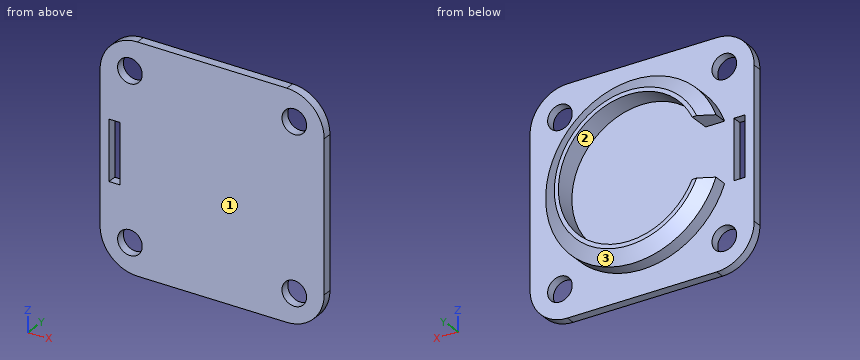
from build123d import *

# Parameters (mm, degrees)
SKETCH2_R           = 11.75
BOSS_EXTRUDE1_DEPTH = 4
CUT_EXTRUDE1_DEPTH  = 4
SKETCH4_W           = 30
SKETCH4_H           = 30
SKETCH4_R           = 1.65
BOSS_EXTRUDE2_DEPTH = 1.2
FILLET2_R           = 5
SKETCH6_W           = 1.5
SKETCH6_H           = 8
CUT_EXTRUDE2_DEPTH  = 10
CHAMFER1_SIZE       = 1
CHAMFER1_SIZE2      = 1.804047755


with BuildPart() as part:
    # Sketch2 → Boss-Extrude1 (new body)
    with BuildSketch(Plane(origin=(0, 0, 0), x_dir=(1, 0, 0), z_dir=(0, 1, 0))):
        with Locations(Location((0, 0, 0), (0, 0, 270))):
            Circle(SKETCH2_R)
    extrude(amount=BOSS_EXTRUDE1_DEPTH)

    # Sketch3 → Cut-Extrude1 (cut)
    with BuildSketch(Plane(origin=(0, 4, 0), x_dir=(1, 0, 0), z_dir=(0, 1, 0))):
        with BuildLine():
            Line((-8.506468127, 4), (-15.473450434, 4))
            Line((-15.473450434, 4), (-15.473450434, -4))
            Line((-15.473450434, -4), (-8.506468127, -4))
            ThreePointArc((-8.506468127, -4), (9.4, 0), (-8.506468127, 4))
        make_face()
    extrude(amount=-CUT_EXTRUDE1_DEPTH, mode=Mode.SUBTRACT)

    # Sketch4 → Boss-Extrude2 (add)
    with BuildSketch(Plane(origin=(0, 0, 0), x_dir=(1, 0, 0), z_dir=(0, 1, 0))):
        Rectangle(SKETCH4_W, SKETCH4_H)
        with Locations(Location((11, -11, 0), (0, 0, 270))):
            Circle(SKETCH4_R, mode=Mode.SUBTRACT)
        with Locations(Location((-11, -11, 0), (0, 0, 270))):
            Circle(SKETCH4_R, mode=Mode.SUBTRACT)
        with Locations(Location((-11, 11, 0), (0, 0, 270))):
            Circle(SKETCH4_R, mode=Mode.SUBTRACT)
        with Locations(Location((11, 11, 0), (0, 0, 270))):
            Circle(SKETCH4_R, mode=Mode.SUBTRACT)
    extrude(amount=BOSS_EXTRUDE2_DEPTH)

    # Fillet2
    fillet2_edges = [part.edges().sort_by_distance(p)[0] for p in [
        (15, 0.6, 15),
        (15, 0.6, -15),
        (-15, 0.6, -15),
        (-15, 0.6, 15),
    ]]
    fillet(fillet2_edges, radius=FILLET2_R)

    # Sketch6 → Cut-Extrude2 (cut)
    with BuildSketch(Plane(origin=(0, 0, 0), x_dir=(1, 0, 0), z_dir=(0, 1, 0))):
        with Locations((-13.05, 0)):
            Rectangle(SKETCH6_W, SKETCH6_H)
    extrude(amount=CUT_EXTRUDE2_DEPTH, mode=Mode.SUBTRACT)

    # Chamfer1
    chamfer1_edges = [part.edges().sort_by_distance(p)[0] for p in [
        (11.75, 4, 0),
    ]]
    chamfer1_side = [part.faces().sort_by_distance(p)[0] for p in [
        (11.75, 2.6, 0),
    ]]
    chamfer(chamfer1_edges, length=CHAMFER1_SIZE, length2=CHAMFER1_SIZE2, reference=chamfer1_side[0])


solid = part.part
Geometry: final body of the model. Coordinates: model frame, mm. Face numbers are marked on the shaded views. Coordinates: 2 decimals unless noted, no trailing zeros. Order: outer loops, then holes, each group sorted by start corner. A loop starts at its lowest first (then second) coordinate and runs counter-clockwise, first axis right, second up.
1) Section C-C (x = 0). Return loops of the section in (y, z).
Result sheet:
outline: (0, -15) - (1.2, -15) - (1.2, -11.75) - (3, -11.75) - (4, -9.95) - (4, -9.4) - (1.2, -9.4) - (1.2, 9.4) - (4, 9.4) - (4, 9.95) - (3, 11.75) - (1.2, 11.75) - (1.2, 15) - (0, 15) - close
2) First-contact query: P1, Ø0.6, axis at x = -13.5, y = 0.5, coming from the -Z side; P2, Ø3, axis at x = -4.5, z = 1, coming from the +Y side; P3, Ø1.3, axis at x = -10, y = 3, coming from the -Z side. Flat tips, straight axial feed; report the tip coordinate or a pass-through.
Result sheet:
P1: stops at z = -13.84
P2: stops at y = 1.2
P3: stops at z = -7.12
3) Section B-B (y = 0.85). Return loops of the section in (x, z).
Result sheet:
outline: (-15, -10) arc R5 ccw to (-10, -15) - (10, -15) arc R5 ccw to (15, -10) - (15, 10) arc R5 ccw to (10, 15) - (-10, 15) arc R5 ccw to (-15, 10) - close; hole (-13.8, -4) - (-12.3, -4) - (-12.3, 4) - (-13.8, 4) - close; hole circle Ø3.3 at (-11, -11); hole circle Ø3.3 at (-11, 11); hole circle Ø3.3 at (11, -11); hole circle Ø3.3 at (11, 11)
4) Draft query along X for the marked faces 1, 2 and 3. Return one class per face: released by +X, released by -X, zero draft, split by the parting line, or undercut.
Result sheet:
face 1: zero draft
face 2: undercut
face 3: split by the parting line
5) Ray query, probe 1 along X at (y, z) = (0.3, 10.75); probe 2 along Y at (x, z) = (8.25, -1); probe 3 along Z at (x, y) = (0, 2.1). Return the intervals inside material, ascending.
Result sheet:
probe 1: x = -14.94 to -12.63, -9.37 to 9.37, 12.63 to 14.94
probe 2: y = 0 to 1.2
probe 3: z = -11.75 to -9.4, 9.4 to 11.75
6) Section A-A (z = 0). Return loops of the section in (x, y), then the cut area to 3 significant figures.
Result sheet:
outline: (-15, 0) - (-13.8, 0) - (-13.8, 1.2) - (-15, 1.2) - close; (-12.3, 0) - (15, 0) - (15, 1.2) - (11.75, 1.2) - (11.75, 3) - (9.95, 4) - (9.4, 4) - (9.4, 1.2) - (-12.3, 1.2) - close
area: 39.9 mm2
7) Section D-D (z = 11). Give the number of separate pieces and of enclosed holes in the cut face, then the cut area to 3 significant figures.
Result sheet:
separate pieces: 3
enclosed holes: 0
area: 45.0 mm2
